from build123d import *

# Parameters (mm, degrees)
SKETCH1_R           = 3.175
BOSS_EXTRUDE1_DEPTH = 3.175
SKETCH1_3_R         = 3.175
BOSS_EXTRUDE2_DEPTH = 3.175
FILLET1_R           = 2.54


with BuildPart() as part:
    # Sketch1 → Boss-Extrude1 (new body)
    with BuildSketch(Plane(origin=(0, 0, 0), x_dir=(1, 0, 0), z_dir=(0, 1, 0))):
        with BuildLine():
            ThreePointArc((3.175, 12.296722124), (0, 12.7), (-3.175, 12.296722124))
            ThreePointArc((-3.175, 12.296722124), (-6.940246952, 6.940246952), (-12.296722124, 3.175))
            ThreePointArc((-12.296722124, 3.175), (-12.7, 0), (-12.296722124, -3.175))
            ThreePointArc((-12.296722124, -3.175), (-6.940246952, -6.940246952), (-3.175, -12.296722124))
            ThreePointArc((-3.175, -12.296722124), (0, -12.7), (3.175, -12.296722124))
            ThreePointArc((3.175, -12.296722124), (6.940246952, -6.940246952), (12.296722124, -3.175))
            ThreePointArc((12.296722124, -3.175), (12.7, 0), (12.296722124, 3.175))
            ThreePointArc((12.296722124, 3.175), (6.940246952, 6.940246952), (3.175, 12.296722124))
        make_face()
        Circle(SKETCH1_R, mode=Mode.SUBTRACT)
    extrude(amount=BOSS_EXTRUDE1_DEPTH)

    # Sketch1_3 → Boss-Extrude2 (add)
    with BuildSketch(Plane(origin=(0, 0, 0), x_dir=(1, 0, 0), z_dir=(0, 1, 0))):
        with BuildLine():
            ThreePointArc((3.175, 5.499261314), (0, 6.35), (-3.175, 5.499261314))
            ThreePointArc((-3.175, 5.499261314), (-4.490128061, 4.490128061), (-5.499261314, 3.175))
            ThreePointArc((-5.499261314, 3.175), (-6.35, 0), (-5.499261314, -3.175))
            ThreePointArc((-5.499261314, -3.175), (-4.490128061, -4.490128061), (-3.175, -5.499261314))
            ThreePointArc((-3.175, -5.499261314), (0, -6.35), (3.175, -5.499261314))
            ThreePointArc((3.175, -5.499261314), (4.490128061, -4.490128061), (5.499261314, -3.175))
            ThreePointArc((5.499261314, -3.175), (6.133628997, -1.643500936), (6.35, 0))
            ThreePointArc((6.35, 0), (6.133628997, 1.643500936), (5.499261314, 3.175))
            ThreePointArc((5.499261314, 3.175), (4.490128061, 4.490128061), (3.175, 5.499261314))
        make_face()
        Circle(SKETCH1_3_R, mode=Mode.SUBTRACT)
    extrude(amount=-BOSS_EXTRUDE2_DEPTH)

    # Fillet1
    fillet1_edges = [part.edges().sort_by_distance(p)[0] for p in [
        (3.175, 1.5875, -12.296722124),
        (12.296722124, 1.5875, -3.175),
        (12.296722124, 1.5875, 3.175),
        (3.175, 1.5875, 12.296722124),
        (-3.175, 1.5875, 12.296722124),
        (-12.296722124, 1.5875, 3.175),
        (-12.296722124, 1.5875, -3.175),
        (-3.175, 1.5875, -12.296722124),
    ]]
    fillet(fillet1_edges, radius=FILLET1_R)


solid = part.part
Geometry check sheet. Reference: the model listing, model coordinates, mm. Give positions to 0.01 mm unless a question says otherwise; leave off trailing zeros. Loops run counter-clockwise (first coordinate to the right, second up) from the corner with the lowest first, then second, coordinate; pieces in that order, holes last.
(1) Release check for a two-part mould opening along X. For faces 1 (the flat face through (-6, 0, 3)), 2 (the cylindrical face through (-0.69, -0.04, 3.1)), 3 (the cylindrical face through (0, 1.6, 12.7)) record: released by +X, released by -X, zero draft, split by the parting line, or undercut.
From the geometry:
face 1: zero draft
face 2: undercut
face 3: split by the parting line
(2) Section check C-C on z = 8.75. Record the cut outline in (x, y) (3 decimals), then the cut area to 3 significant figures.
From the geometry:
outline: (-5.346, 0) - (5.346, 0) - (5.346, 3.175) - (-5.346, 3.175) - close
area: 33.9 mm2
(3) Depth check by flat-ended pin: pin 1 Ø1 at (x, y) = (2.5, -2.5) entering from +Z; pin 2 Ø2 at (x, y) = (2.5, 1) entering from +Z. Enter the tip coordinate at first touch or a pass-through.
From the geometry:
pin 1: stops at z = 6.03
pin 2: stops at z = 12.61
(4) Thickness scan on L1, parallel to X at y = -1.5, z = 0 (3 decimals); L2, parallel to Y at x = -10, z = 1.5 (3 decimals). Record the ranges inside material, lowest first.
From the geometry:
L1: x = -6.35 to -3.175, 3.175 to 6.35
L2: y = 0 to 3.175
(5) Section check B-B on y = -0.75. Record the cut outline in (x, z) (3 decimals).
From the geometry:
outline: circle Ø12.7 at (0, 0); hole circle Ø6.35 at (0, 0)
(6) Section check A-A on x = 0. Record the cut outline in (y, z) (3 decimals), then the cut area to 3 significant figures.
From the geometry:
outline: (-3.175, -6.35) - (0, -6.35) - (0, -12.7) - (3.175, -12.7) - (3.175, -3.175) - (-3.175, -3.175) - close; (-3.175, 3.175) - (3.175, 3.175) - (3.175, 12.7) - (0, 12.7) - (0, 6.35) - (-3.175, 6.35) - close
area: 80.6 mm2
(7) Section check D-D on x = 10.5. Record the cut outline in (y, z) (3 decimals).
From the geometry:
outline: (0, -4.142) - (3.175, -4.142) - (3.175, 4.142) - (0, 4.142) - close
